from build123d import *

# Parameters (mm, degrees)
F0_R     = 987.425
F0_R_2   = 981.075
F1_DEPTH = 609.6
F2_R     = 44.45
F3_DEPTH = 987.426


with BuildPart() as f1:
    # F0 (on Top) → F1 (new body)
    with BuildSketch(Plane.XY):
        Circle(F0_R)
        Circle(F0_R_2, mode=Mode.SUBTRACT)
    extrude(amount=F1_DEPTH)

    # F2 (on Front) → F3 (cut, through all)
    with BuildSketch(Plane.XZ):
        with Locations((-949.452, 444.5)):
            Circle(F2_R)
        with Locations((-949.452, 165.1)):
            Circle(F2_R)
    extrude(amount=F3_DEPTH, mode=Mode.SUBTRACT)


solid = f1.part
Input: part model. Units: mm. Frame: model coordinates. Coordinates: 2 decimals unless noted, no trailing zeros. Loops run counter-clockwise (first coordinate to the right, second up) from the corner with the lowest first, then second, coordinate; pieces in that order, holes last. Notation, with made-up numbers: (32.5, 36) -> (72.5, 36) arc R20 ccw to (72.5, 51) -> close; hole circle Ø7 at (24.5, -24). An arc over 180 degrees is marked (long way). One line per item, written item: value.
(1) Ray query, line 1 along Y through (x, z) = (0, 325) (3 decimals); line 2 along X through (y, z) = (24, 477); line 3 along X through (y, z) = (-21.5, 359.5). Return the intervals inside material, ascending.
Answer below:
line 1: y = -987.425 to -981.075, 981.075 to 987.425
line 2: x = -987.13 to -980.78, 980.78 to 987.13
line 3: x = -987.19 to -980.84, 980.84 to 987.19
(2) Draft query along Y for faces 1 (the face through (-214.054, -963.944, 300.533)), 2 (the face through (452.71, -870.38, 300.53)). Return one class per face: pulls with the +Y half, pulls with the -Y half, needs draft (parallel to the pull), parting line crosses it, or undercut.
Answer below:
face 1: parting line crosses it
face 2: undercut
(3) Cut plane A-A (x = 0). Output: boundary loops of the cut face in (y, z) (3 decimals), then the cut area to 3 significant figures.
Answer below:
outline: (-987.425, 0) -> (-981.075, 0) -> (-981.075, 609.6) -> (-987.425, 609.6) -> close; (981.075, 0) -> (987.425, 0) -> (987.425, 609.6) -> (981.075, 609.6) -> close
area: 7,740 mm2
(4) Cut plane C-C (z = 239.5). Output: boundary loops of the cut face in (x, y) (3 decimals), then the cut area to 3 significant figures.
Answer below:
outline: circle Ø1974.85 at (0, 0); hole circle Ø1962.15 at (0, 0)
area: 39,300 mm2
(5) Pin query (flat end, axial travel): pin 1 Ø5 at (x, z) = (-983, 166) entering from -Y; pin 2 Ø4 at (x, z) = (562.5, 524) entering from +Y; pin 3 Ø8 at (x, z) = (-588.5, 453.5) entering from -Y. Return the tip coordinate at first contact, or that it passes through.
Answer below:
pin 1: stops at y = 0
pin 2: stops at y = 812.93
pin 3: stops at y = -795.84
